Here's how the part is built. I have some questions about the finished solid (model axes, mm). Face numbers are marked on the shaded views. A direction names the side the tool comes from. Coordinates: 2 decimals unless noted, no trailing zeros. Loops run counter-clockwise (first coordinate to the right, second up) from the corner with the lowest first, then second, coordinate; pieces in that order, holes last. Notation, with made-up numbers: (-10, 41) - (29, 41) arc R16 cw to (29, 63) - close; hole circle Ø11 at (59, -14). An arc over 180 degrees is marked (long way). Use a Markdown table: item, result.
```python
from build123d import *

# Parameters (mm, degrees)
F1_DEPTH = 1.5875
F2_COUNT = 16
F0_R     = 1.5875
F3_DEPTH = 1.5875
F4_DEPTH = 12.7


with BuildPart() as f1:
    # F0 (on Top) → F1 (new body)
    with BuildSketch(Plane.XY):
        with BuildLine():
            ThreePointArc((-1.0511033425, 4.8401849927), (-0.4854788961, 4.9291499512), (0.0866334376, 4.9522422848))
            ThreePointArc((0.0866334376, 4.9522422848), (0.0809330254, 5.2752470416), (0, 5.588))
            ThreePointArc((0, 5.588), (-0.2484578592, 6.0002980681), (-0.6210025483, 6.3051446843))
            ThreePointArc((-0.6210025483, 6.3051446843), (-0.9269162712, 5.933475747), (-1.0901647194, 5.4806281469))
            ThreePointArc((-1.0901647194, 5.4806281469), (-1.1085275641, 5.1580953989), (-1.0511033425, 4.8401849927))
        make_face()
    extrude(amount=F1_DEPTH)


with BuildPart() as f2_1:
    # F2: instance of F1
    add(f1.part.rotate(Axis((0, 0, 0), (0, 0, 1)), 1 * 360 / F2_COUNT))


with BuildPart() as f2_2:
    # F2: instance of F1
    add(f1.part.rotate(Axis((0, 0, 0), (0, 0, 1)), 2 * 360 / F2_COUNT))


with BuildPart() as f2_3:
    # F2: instance of F1
    add(f1.part.rotate(Axis((0, 0, 0), (0, 0, 1)), 3 * 360 / F2_COUNT))


with BuildPart() as f2_4:
    # F2: instance of F1
    add(f1.part.rotate(Axis((0, 0, 0), (0, 0, 1)), 4 * 360 / F2_COUNT))


with BuildPart() as f2_5:
    # F2: instance of F1
    add(f1.part.rotate(Axis((0, 0, 0), (0, 0, 1)), 5 * 360 / F2_COUNT))


with BuildPart() as f2_6:
    # F2: instance of F1
    add(f1.part.rotate(Axis((0, 0, 0), (0, 0, 1)), 6 * 360 / F2_COUNT))


with BuildPart() as f2_7:
    # F2: instance of F1
    add(f1.part.rotate(Axis((0, 0, 0), (0, 0, 1)), 7 * 360 / F2_COUNT))


with BuildPart() as f2_8:
    # F2: instance of F1
    add(f1.part.rotate(Axis((0, 0, 0), (0, 0, 1)), 8 * 360 / F2_COUNT))


with BuildPart() as f2_9:
    # F2: instance of F1
    add(f1.part.rotate(Axis((0, 0, 0), (0, 0, 1)), 9 * 360 / F2_COUNT))


with BuildPart() as f2_10:
    # F2: instance of F1
    add(f1.part.rotate(Axis((0, 0, 0), (0, 0, 1)), 10 * 360 / F2_COUNT))


with BuildPart() as f2_11:
    # F2: instance of F1
    add(f1.part.rotate(Axis((0, 0, 0), (0, 0, 1)), 11 * 360 / F2_COUNT))


with BuildPart() as f2_12:
    # F2: instance of F1
    add(f1.part.rotate(Axis((0, 0, 0), (0, 0, 1)), 12 * 360 / F2_COUNT))


with BuildPart() as f2_13:
    # F2: instance of F1
    add(f1.part.rotate(Axis((0, 0, 0), (0, 0, 1)), 13 * 360 / F2_COUNT))


with BuildPart() as f2_14:
    # F2: instance of F1
    add(f1.part.rotate(Axis((0, 0, 0), (0, 0, 1)), 14 * 360 / F2_COUNT))


with BuildPart() as f2_15:
    # F2: instance of F1
    add(f1.part.rotate(Axis((0, 0, 0), (0, 0, 1)), 15 * 360 / F2_COUNT))


with BuildPart() as f1_1:
    add(f1.part)

    add(f2_1.part)  # F3 merges F2_1

    add(f2_2.part)  # F3 merges F2_2

    add(f2_3.part)  # F3 merges F2_3

    add(f2_4.part)  # F3 merges F2_4

    add(f2_5.part)  # F3 merges F2_5

    add(f2_6.part)  # F3 merges F2_6

    add(f2_7.part)  # F3 merges F2_7

    add(f2_8.part)  # F3 merges F2_8

    add(f2_9.part)  # F3 merges F2_9

    add(f2_10.part)  # F3 merges F2_10

    add(f2_11.part)  # F3 merges F2_11

    add(f2_12.part)  # F3 merges F2_12

    add(f2_13.part)  # F3 merges F2_13

    add(f2_14.part)  # F3 merges F2_14

    add(f2_15.part)  # F3 merges F2_15
    # F0 (on Top) → F3 (join)
    with BuildSketch(Plane.XY):
        with BuildLine():
            ThreePointArc((-1.0511033425, 4.8401849927), (-3.1085442047, -3.8560552288), (4.953, 0))
            ThreePointArc((4.953, 0), (3.5327966554, 3.4715352211), (0.0866334376, 4.9522422848))
            ThreePointArc((0.0866334376, 4.9522422848), (-0.4854788961, 4.9291499512), (-1.0511033425, 4.8401849927))
        make_face()
        Circle(F0_R, mode=Mode.SUBTRACT)
    extrude(amount=F3_DEPTH)

    # F0 (on Top) → F4 (join)
    with BuildSketch(Plane.XY):
        Circle(F0_R)
    extrude(amount=F4_DEPTH)


solid = f1_1.part
```
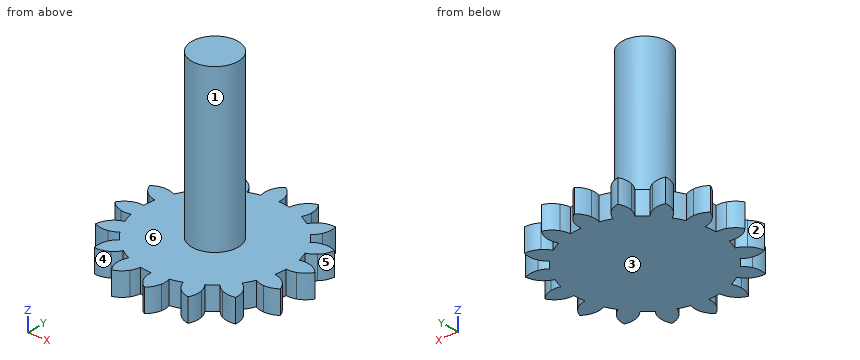
Q1. I want a section at A-A, the plane x = -3.75. Write out the boundary of the cut face in (y, z), then the cut area to 3 significant figures.
Check values:
| item | result |
|---|---|
| outline | (-4.89, 0) - (-3.63, 0) - (-3.63, 1.59) - (-4.89, 1.59) - close; (-3.24, 0) - (3.84, 0) - (3.84, 1.59) - (-3.24, 1.59) - close |
| area | 13.2 mm^2 |
Q2. Which directions (+Z, -Z, +X, -X, +Y, -Y) give clear straight access to the entire face, cutting with the end or side of a thin tool? Please do the marked faces 1, 2 and 3.
Check values:
| item | result |
|---|---|
| face 1 | +Z |
| face 2 | +Z, -Z, -X |
| face 3 | -Z, +X, -X, +Y, -Y |
Q3. If we mould it in two halves opening along X, with no side actions, what happens to the marked faces 4, 5 and 6? For each: pulls with the +X half, pulls with the -X half, needs draft (parallel to the pull), parting line crosses it, or undercut.
Check values:
| item | result |
|---|---|
| face 4 | undercut |
| face 5 | pulls with the +X half |
| face 6 | needs draft |
Q4. Please list where these lines run through material, in increasing order: L1, parallel to Z at x = -3, y = -3.5; L2, parallel to Y at x = 0, z = 5; L3, parallel to Y at x = -1, z = 5. Write a range as from..to.
Check values:
| item | result |
|---|---|
| L1 | 0..1.59 |
| L2 | -1.59..1.59 |
| L3 | -1.23..1.23 |
Q5. Will these pins go through, and if not, where does the flat tip stop? P1, Ø3, axis at x = 1.5, z = 4, coming from the +Y side; P2, Ø4, axis at x = 1, z = 6.5, coming from the -Y side; P3, Ø5, axis at x = 3.5, z = 11, coming from the -Y side.
Check values:
| item | result |
|---|---|
| P1 | y = 1.59 |
| P2 | y = -1.59 |
| P3 | y = -1.23 |
Q6. I want a section at B-B, the plane z = 8. Write out the boundary of the cut face in (x, y) (1 decimal), then the cut area to 3 significant figures.
Check values:
| item | result |
|---|---|
| outline | circle Ø3.2 at (0, 0) |
| area | 7.92 mm^2 |
